Input: part model. Units: mm. Frame: model coordinates. A direction names the side the tool comes from. Round coordinates to 2 decimals unless told otherwise and drop trailing zeros. Order: outer loops, then holes, each group sorted by start corner. A loop starts at its lowest first (then second) coordinate and runs counter-clockwise, first axis right, second up. Notation, with made-up numbers: M -6.75,-33.75 L 14.25,-33.75 A31 cw 14.25,4.25 Z; hole C 70,70.5 d8. An arc over 180 degrees is marked long. One line per question, with ' | ' between items.
```python
from build123d import *

# Parameters (mm, degrees)
EXTRUDE_1_DEPTH          = 10
EXTRUDE_1_DEPTH_BACK     = 20
SKETCH_1_W               = 550
SKETCH_1_H               = 900
CUT_EXTRUDE_4_DEPTH      = 20
SKETCH_7_R               = 50
CUT_EXTRUDE_5_DEPTH      = 5
SKETCH_8_W               = 25
SKETCH_8_H               = 25
EXTRUDE_2_DEPTH          = 30
SKETCH_9_R               = 8
CUT_EXTRUDE_6_DEPTH      = 5
SKETCH_10_R              = 8
CUT_EXTRUDE_7_DEPTH      = 5
MIRROR_2_COPY_1_SKETCH_W = 25
MIRROR_2_COPY_1_SKETCH_H = 25
MIRROR_2_COPY_1_DEPTH    = 30
MIRROR_2_COPY_2_SKETCH_R = 8
MIRROR_2_COPY_2_DEPTH    = 5
MIRROR_2_COPY_3_SKETCH_R = 8
MIRROR_2_COPY_3_DEPTH    = 5


with BuildPart() as part:
    # 草图1 → 凸台-拉伸1 (new, two sides: drawn at the far end of the back side and taken through both)
    with BuildSketch(Plane(origin=(0, 0, 0), x_dir=(1, 0, 0), z_dir=(0, 1, 0)).offset(-EXTRUDE_1_DEPTH_BACK)):
        Rectangle(SKETCH_1_W, SKETCH_1_H)
    extrude(amount=EXTRUDE_1_DEPTH + EXTRUDE_1_DEPTH_BACK)

    # 草图6 → 切除-拉伸4 (cut)
    with BuildSketch(Plane(origin=(0, 10, 0), x_dir=(1, 0, 0), z_dir=(0, 1, 0))):
        with BuildLine():
            Line((-150.934743828, 363.792707869), (150.934743828, 363.792707869))
            ThreePointArc((150.934743828, 363.792707869), (172.147947264, 355.005911305), (180.934743828, 333.792707869))
            Line((180.934743828, 333.792707869), (180.934743828, -333.792707869))
            ThreePointArc((180.934743828, -333.792707869), (172.147947264, -355.005911305), (150.934743828, -363.792707869))
            Line((150.934743828, -363.792707869), (-150.934743828, -363.792707869))
            ThreePointArc((-150.934743828, -363.792707869), (-172.147947264, -355.005911305), (-180.934743828, -333.792707869))
            Line((-180.934743828, -333.792707869), (-180.934743828, 333.792707869))
            ThreePointArc((-180.934743828, 333.792707869), (-172.147947264, 355.005911305), (-150.934743828, 363.792707869))
        make_face()
    extrude(amount=-CUT_EXTRUDE_4_DEPTH, mode=Mode.SUBTRACT)

    # 草图7 → 切除-拉伸5 (cut)
    with BuildSketch(Plane.XZ.offset(20)):
        with Locations(Location((-215, 300, 0), (0, 0, 270))):
            Circle(SKETCH_7_R)
        with Locations(Location((-215, -300, 0), (0, 0, 90))):
            Circle(SKETCH_7_R)
        with Locations(Location((215, -300, 0), (0, 0, 270))):
            Circle(SKETCH_7_R)
        with Locations(Location((215, 300, 0), (0, 0, 90))):
            Circle(SKETCH_7_R)
    extrude(amount=-CUT_EXTRUDE_5_DEPTH, mode=Mode.SUBTRACT)

    # 草图8 → 凸台-拉伸2 (add)
    with BuildSketch(Plane.XZ.offset(20)):
        with Locations((-262.5, -462.5)):
            Rectangle(SKETCH_8_W, SKETCH_8_H)
        with Locations((-287.5, -437.5)):
            Rectangle(SKETCH_8_W, SKETCH_8_H)
    extrude_2 = extrude(amount=-EXTRUDE_2_DEPTH)

    # 草图9 → 切除-拉伸6 (cut)
    with BuildSketch(Plane.ZY.offset(300)):
        with Locations((-437.5, -5)):
            Circle(SKETCH_9_R)
    cut_extrude_6 = extrude(amount=-CUT_EXTRUDE_6_DEPTH, mode=Mode.SUBTRACT)

    # 草图10 → 切除-拉伸7 (cut)
    with BuildSketch(Plane(origin=(0, 0, -475), x_dir=(-1, 0, 0), z_dir=(0, 0, -1))):
        with Locations((262.5, -5)):
            Circle(SKETCH_10_R)
    cut_extrude_7 = extrude(amount=-CUT_EXTRUDE_7_DEPTH, mode=Mode.SUBTRACT)

    # 镜向1: 凸台-拉伸2, 切除-拉伸6, 切除-拉伸7 across plane
    add(extrude_2.mirror(Plane(origin=(0, 0, 0), x_dir=(0, 0, 1), z_dir=(1, 0, 0))))
    add(cut_extrude_6.mirror(Plane(origin=(0, 0, 0), x_dir=(0, 0, 1), z_dir=(1, 0, 0))), mode=Mode.SUBTRACT)
    add(cut_extrude_7.mirror(Plane(origin=(0, 0, 0), x_dir=(0, 0, 1), z_dir=(1, 0, 0))), mode=Mode.SUBTRACT)

    # 镜向2: 凸台-拉伸2, 切除-拉伸6, 切除-拉伸7 across plane
    add(extrude_2.mirror(Plane.XY))
    add(cut_extrude_6.mirror(Plane.XY), mode=Mode.SUBTRACT)
    add(cut_extrude_7.mirror(Plane.XY), mode=Mode.SUBTRACT)

    # 镜向2 copy 1 sketch → 镜向2 copy 1 (add)
    with BuildSketch(Plane(origin=(0, -20, 0), x_dir=(-1, 0, 0), z_dir=(0, -1, 0))):
        with Locations((-262.5, -462.5)):
            Rectangle(MIRROR_2_COPY_1_SKETCH_W, MIRROR_2_COPY_1_SKETCH_H)
        with Locations((-287.5, -437.5)):
            Rectangle(MIRROR_2_COPY_1_SKETCH_W, MIRROR_2_COPY_1_SKETCH_H)
    extrude(amount=-MIRROR_2_COPY_1_DEPTH)

    # 镜向2 copy 2 sketch → 镜向2 copy 2 (cut)
    with BuildSketch(Plane(origin=(300, 0, 0), x_dir=(0, 0, -1), z_dir=(1, 0, 0))):
        with Locations((-437.5, -5)):
            Circle(MIRROR_2_COPY_2_SKETCH_R)
    extrude(amount=-MIRROR_2_COPY_2_DEPTH, mode=Mode.SUBTRACT)

    # 镜向2 copy 3 sketch → 镜向2 copy 3 (cut)
    with BuildSketch(Plane.XY.offset(475)):
        with Locations((262.5, -5)):
            Circle(MIRROR_2_COPY_3_SKETCH_R)
    extrude(amount=-MIRROR_2_COPY_3_DEPTH, mode=Mode.SUBTRACT)


solid = part.part
```
Item 1: Section query A-A, the plane x = -215. Return loops of the section in (y, z), plus the area to 3 significant figures.
Report:
outline: M -20,-450 L 10,-450 L 10,450 L -20,450 L -20,350 L -15,350 L -15,250 L -20,250 L -20,-250 L -15,-250 L -15,-350 L -20,-350 Z | area: 26,000 mm²
Item 2: Access query for faces 1 (the flat face through (288, -5, 425)), 2 (the flat face through (288, -5, 450)), 3 (the cylindrical face through (165.425, -17.535, 293.491)). Directions: +Z, -Z, +X, -X, +Y, -Y. A direction counts if a zero-diameter tool reaches every point of the face in a straight line with its end or side. Return the directions, or none.
Report:
face 1: +X, +Y, -Y | face 2: +Z, +X, +Y, -Y | face 3: -Y
Item 3: Section query B-B, the plane z = 300. Return loops of the section in (x, y), plus the area to 3 significant figures.
Report:
outline: M -275,-20 L -265,-20 L -265,-15 L -165,-15 L -165,-20 L 165,-20 L 165,-15 L 265,-15 L 265,-20 L 275,-20 L 275,10 L 180.93,10 L 180.93,-10 L -180.93,-10 L -180.93,10 L -275,10 Z | area: 8,260 mm²
Item 4: Section query C-C, the plane x = -120. Return loops of the section in (y, z).
Report:
outline: M -20,-450 L 10,-450 L 10,-363.79 L -10,-363.79 L -10,363.79 L 10,363.79 L 10,450 L -20,450 Z
Item 5: Section query D-D, the plane z = -182. Return loops of the section in (x, y).
Report:
outline: M -275,-20 L 275,-20 L 275,10 L 180.93,10 L 180.93,-10 L -180.93,-10 L -180.93,10 L -275,10 Z
Item 6: Line query: line 1 along X through (y, z) = (-16.1, 300); line 2 along X through (y, z) = (-6, -171.5); line 3 along Y through (x, z) = (-298.65, -437.5). Output: solid intervals per line, ascending. Write a range as from..to.
Report:
line 1: -275..-265, -165..165, 265..275 | line 2: -275..-180.93, 180.93..275 | line 3: -20..-13, 3..10
Item 7: Mould query, pull axis X, two halves, no side actions, for faces 4 (the flat face through (-275, -5, 6)), 5 (the flat face through (275, -5, 6)), 6 (the flat face through (250, -5, -463)), 7 (the flat face through (288, -5, -450)). Classes: +X half, -X half, draft (parallel to the pull), parting line (faces both ways), or undercut.
Report:
face 4: -X half | face 5: +X half | face 6: undercut | face 7: draft
Item 8: First-contact query: pin 1 (1.5 mm diameter, centred on x = 80, y = 1, fed in from +Z); pin 2 (6 mm diameter, centred on y = -12.5, z = -296.5, fed in from -X); pin 3 (1.5 mm diameter, centred on x = -215.5, z = -344.5, fed in from -Y); pin 4 (17.5 mm diameter, centred on x = 264.5, y = -5, fed in from -Z). Flat tips, straight axial feed; report the tip coordinate or a pass-through.
Report:
pin 1: z = 450 | pin 2: x = -275 | pin 3: y = -15 | pin 4: z = -475
